Input: part model. Units: mm. Frame: model coordinates. Face numbers are marked on the shaded views. A direction names the side the tool comes from. Give positions to 0.01 mm unless a question says otherwise; leave off trailing zeros. Loops run counter-clockwise (first coordinate to the right, second up) from the corner with the lowest first, then second, coordinate; pieces in that order, holes last. Notation, with made-up numbers: M 86,48 L 125,48 A17 cw 125,55 Z; hole C 5,-19.75 d7. An arc over 180 degrees is marked long. One line per item, written item: value. Start each with the question number.
(1) Ray query, line 1 along Y through (x, z) = (-39, 2.5); line 2 along X through (y, z) = (54, 9); line 3 along Y through (x, z) = (28.5, 9). Return the intervals inside material, ascending. Write a range as from..to.
(2) Pull-direction query (Y, two-part tool) for the marked faces 4, 5, 6 and 7; classes: released by +Y, released by -Y, zero draft, split by the parting line, or undercut.
(3) Access query for the marked faces 1, 2 and 3. Directions: +Z, -Z, +X, -X, +Y, -Y. A direction counts if a zero-diameter tool reaches every point of the face in a straight line with its end or side. Return the directions, or none.
(4) Section A-A on x = -8. Output: boundary loops of the cut face in (y, z), plus the area to 3 significant figures.
(5) Section B-B on y = 83.5. Output: boundary loops of the cut face in (x, z), plus the area to 3 significant figures.
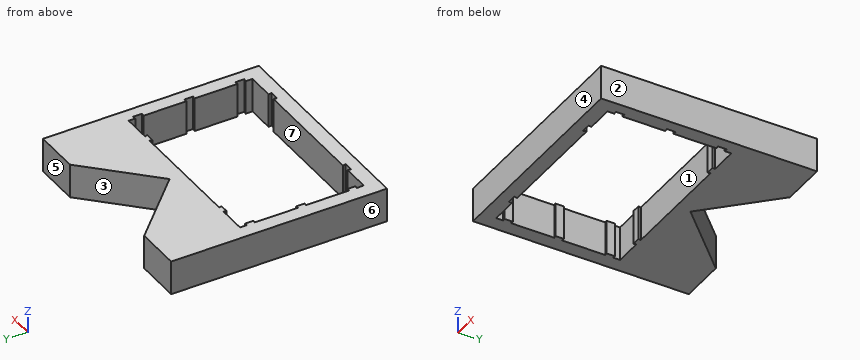
```python
from build123d import *

# Parameters (mm, degrees)
PAD_DEPTH = 15


with BuildPart() as part:
    # Sketch → Pad (new body)
    with BuildSketch(Plane.XY):
        Polygon((0, 67.5), (-27.5, 95), (-47.5, 95), (-47.5, 0), (47.5, 0), (47.5, 95), (27.5, 95), align=None)
        Polygon((-41.25, 61), (-29.15, 61), (-29.4, 59.8), (-25.6, 59.8), (-25.85, 61), (25.85, 61), (25.6, 59.8), (29.4, 59.8), (29.15, 61), (41.25, 61), (41.25, 58), (42.65, 58.25), (42.65, 54.25), (41.25, 54.5), (41.25, 35.5), (42.65, 35.75), (42.65, 31.75), (41.25, 32), (41.25, 13), (42.65, 13.25), (42.65, 9.25), (41.25, 9.5), (41.25, 6.5), (29.25, 6.5), (29.5, 5.1), (25.5, 5.1), (25.75, 6.5), (-25.75, 6.5), (-25.5, 5.1), (-29.5, 5.1), (-29.25, 6.5), (-41.25, 6.5), (-41.25, 9.6), (-40.05, 9.35), (-40.05, 13.15), (-41.25, 12.9), (-41.25, 32.1), (-40.05, 31.85), (-40.05, 35.65), (-41.25, 35.4), (-41.25, 54.6), (-40.05, 54.35), (-40.05, 58.15), (-41.25, 57.9), align=None, mode=Mode.SUBTRACT)
    extrude(amount=PAD_DEPTH)


solid = part.part
```
Output values:
1. line 1: y = 0..6.5, 61..95
1. line 2: x = -47.5..-41.25, 41.25..47.5
1. line 3: y = 0..5.1, 59.8..95
2. face 4: released by -Y
2. face 5: released by +Y
2. face 6: zero draft
2. face 7: undercut
3. face 1: +Z, -Z
3. face 2: +Z, -Z, +X, +Y, -Y
3. face 3: +Z, -Z, +Y
4. outline: M 0,0 L 6.5,0 L 6.5,15 L 0,15 Z; M 61,0 L 75.5,0 L 75.5,15 L 61,15 Z
4. area: 315 mm²
5. outline: M -47.5,0 L -16,0 L -16,15 L -47.5,15 Z; M 16,0 L 47.5,0 L 47.5,15 L 16,15 Z
5. area: 945 mm²
